```python
from build123d import *

# Parameters (mm, degrees)
F0_R      = 27.8603665739
F1_DEPTH  = 3.048
F4_R      = 26.2786257822
F5_DEPTH  = 1.016
F6_R      = 22.2176168744
F7_DEPTH  = 3.302
F9_R      = 15.773437446
F10_DEPTH = 2.032
F11_R     = 2.2956006308
F12_DEPTH = 21.336
F13_R     = 2.0464830212
F14_DEPTH = 25.4


# Not quite as in the source:
# - a fillet or chamfer that OpenCascade refuses, or shapes differently, is made with other operations: its cross-section is extruded or revolved along the edge and cut away or added


with BuildPart() as f1:
    # F0 (on Top) → F1 (new body)
    with BuildSketch(Plane.XY):
        Circle(F0_R)
    extrude(amount=F1_DEPTH)

    # F2: fillet of radius 5.08 on 1 edges, made by hand

    # F2_s1 → F2_t2 (revolve, cut)
    with BuildSketch(Plane.XZ):
        with BuildLine():
            ThreePointArc((27.8603665739, 0), (25.9869002599, 2.2182329348), (23.2044696678, 3.048))
            Line((23.2044696678, 3.048), (27.8603665739, 3.048))
            Line((27.8603665739, 3.048), (27.8603665739, 0))
        make_face()
    revolve(axis=Axis((0, 0, 3.048), (0, 0, 1)), mode=Mode.SUBTRACT)

    # F4 (on face) → F5 (join)
    with BuildSketch(Plane(origin=(0, 0, 0), x_dir=(1, 0, 0), z_dir=(0, 0, -1))):
        Circle(F4_R)
    extrude(amount=F5_DEPTH)

    # F6 (on face) → F7 (join)
    with BuildSketch(Plane.XY.offset(3.048)):
        Circle(F6_R)
    extrude(amount=F7_DEPTH)

    # F8: fillet of radius 5.08 on 1 edges, made by hand

    # F8_s1 → F8_t2 (revolve, cut)
    with BuildSketch(Plane.XZ):
        with BuildLine():
            ThreePointArc((22.2176168744, 3.048), (20.3549739793, 5.4436458882), (17.4589283996, 6.35))
            Line((17.4589283996, 6.35), (22.2176168744, 6.35))
            Line((22.2176168744, 6.35), (22.2176168744, 3.048))
        make_face()
    revolve(axis=Axis((0, 0, 6.35), (0, 0, 1)), mode=Mode.SUBTRACT)

    # F9 (on face) → F10 (cut)
    with BuildSketch(Plane.XY.offset(6.35)):
        Circle(F9_R)
    extrude(amount=-F10_DEPTH, mode=Mode.SUBTRACT)

    # F11 (on face) → F12 (cut)
    with BuildSketch(Plane.XY.offset(3.048)):
        with Locations((-17.1565320343, -10.5084851384)):
            Circle(F11_R)
    extrude(amount=-F12_DEPTH, mode=Mode.SUBTRACT)

    # F13 (on face) → F14 (cut)
    with BuildSketch(Plane.XY.offset(6.35)):
        with Locations((-17.3885338008, -10.6187639758)):
            Circle(F13_R)
    extrude(amount=-F14_DEPTH, mode=Mode.SUBTRACT)


solid = f1.part
```
Can you work these out from the model? Positions are in its coordinate system, mm. A direction names the side the tool comes from. Give positions to 0.01 mm unless a question says otherwise; leave off trailing zeros. Loops run counter-clockwise (first coordinate to the right, second up) from the corner with the lowest first, then second, coordinate; pieces in that order, holes last. Notation, with made-up numbers: M -0.75,33 L 35.25,33 A24 cw 35.25,69 Z; hole C 67.25,5.5 d2. An arc over 180 degrees is marked long. Use CSV: the item, a comma, the result in double quotes. Start each with the question number.
1. For P1, Ø2, axis at x = 1, z = 3, coming from the +Y side; P2, Ø9.5, axis at x = 2, y = -6, coming from the +Z side; P3, Ø3.5, axis at x = -17.39, y = -10.62, coming from the +Z side; P4, Ø4, axis at x = -10, z = 3.5, coming from the -Y side, each with a flat end and sliding along its axis, tell me the tip position at first contact or that it passes through.
2. Imagine slicing it at C-C, the plane z = 1. Write out the boundary of the cut face in (x, y).
3. If I drill on L1, parallel to X at y = -7.5, z = 4.75; L2, parallel to Z at x = 25, y = 11; L3, parallel to Z at x = -7, y = 11.5, over which ranges is the centre line in solid material (lowest first)?
4. On a 3-axis mill with a long thin cutter (end or side, diameter ignored), from which of +Z, -Z, +X, -X, +Y, -Y can I reach the whole of each face in a straight line? I mean faces 1 (the face through (0, 0, -1.016)), 2 (the face through (19, -12, 3.048)), 3 (the face through (-15.045, -9.608, 1.044)). Say none if no direction works.
5. Imagine slicing it at A-A, the plane x = 0. Write out the boundary of the cut face in (y, z), plus the area to 3 significant figures.
6. If we mould it in two halves opening along X, with no side actions, what happens to faces 4 (the face through (-5.697, 25.654, -0.501)), 5 (the face through (-15.603, -9.618, 4.326)), 6 (the face through (-17, -21, 0))? For each: released by +X, released by -X, zero draft, split by the parting line, or undercut.
Response values:
1,P1,"y = 26.28"
1,P2,"z = 4.32"
1,P3,"through"
1,P4,"y = -25.06"
2,outline,"C 0,0 d54.56; hole M -19.4,-10.99 A2.05 ccw -18.95,-11.94 A2.3 ccw long Z"
3,L1,"-19.79 to -13.88, 13.88 to 19.79"
3,L2,"0 to 0.96"
3,L3,"-1.02 to 4.32"
4,face 1,"-Z, +X, -X, +Y, -Y"
4,face 2,"+Z"
4,face 3,"-Z"
5,outline,"M -27.86,0 L -26.28,0 L -26.28,-1.02 L 26.28,-1.02 L 26.28,0 L 27.86,0 A5.08 ccw 23.2,3.05 L 22.22,3.05 A5.08 ccw 17.46,6.35 L 15.77,6.35 L 15.77,4.32 L -15.77,4.32 L -15.77,6.35 L -17.46,6.35 A5.08 ccw -22.22,3.05 L -23.2,3.05 A5.08 ccw Z"
5,area,"289 mm^2"
6,face 4,"split by the parting line"
6,face 5,"undercut"
6,face 6,"zero draft"
